from build123d import *

# Parameters (mm, degrees)
SKETCH1_W                               = 304.8
SKETCH1_H                               = 304.8
BOSS_EXTRUDE1_DEPTH                     = 38.1
SKETCH2_R                               = 6.5151
HAAS_T_SLOT_HOLES_DEPTH                 = 219.867836833
SKETCH3_R                               = 9.779
HAAS_COUNTER_BORES_DEPTH                = 22.225
SKETCH4_R                               = 6.5151
TORMACH_T_SLOT_HOLES_DEPTH              = 219.867836833
SKETCH5_R                               = 9.779
TORMACH_COUNTER_BORES_DEPTH             = 22.225
SKETCH6_R                               = 3.0734
SPROCKET_LOCATING_HOLES_DEPTH           = 6.35
SKETCH7_R                               = 3.175
SPROCKET_MOUNTING_CLEARANCE_HOLES_DEPTH = 9.525
SKETCH8_R                               = 5.9182
F_1_2_13_TAPPED_HOLES_DEPTH             = 19.05
SKETCH9_R                               = 3.175
SKETCH9_R_2                             = 3.3
SKETCH9_R_3                             = 2.5
SKETCH9_R_4                             = 4.5
CUT_EXTRUDE1_DEPTH                      = 19.05


with BuildPart() as part:
    # Sketch1 → Boss-Extrude1 (new body)
    with BuildSketch(Plane.XY):
        Rectangle(SKETCH1_W, SKETCH1_H)
    extrude(amount=BOSS_EXTRUDE1_DEPTH)

    # Sketch2 → HAAS T-Slot Holes (cut, through all)
    with BuildSketch(Plane.XY.offset(38.1)):
        with Locations((-127, 101.6)):
            Circle(SKETCH2_R)
        with Locations((127, 101.6)):
            Circle(SKETCH2_R)
        with Locations((127, -101.6)):
            Circle(SKETCH2_R)
        with Locations((-127, -101.6)):
            Circle(SKETCH2_R)
        Circle(SKETCH2_R)
    extrude(amount=-HAAS_T_SLOT_HOLES_DEPTH, mode=Mode.SUBTRACT)

    # Sketch3 → HAAS Counter Bores (cut)
    with BuildSketch(Plane.XY.offset(38.1)):
        with Locations((-127, 101.6)):
            Circle(SKETCH3_R)
        with Locations((127, 101.6)):
            Circle(SKETCH3_R)
        Circle(SKETCH3_R)
        with Locations((127, -101.6)):
            Circle(SKETCH3_R)
        with Locations((-127, -101.6)):
            Circle(SKETCH3_R)
    extrude(amount=-HAAS_COUNTER_BORES_DEPTH, mode=Mode.SUBTRACT)

    # Sketch4 → Tormach T-Slot Holes (cut, through all)
    with BuildSketch(Plane.XY.offset(38.1)):
        with Locations((-101.6, 90.4875)):
            Circle(SKETCH4_R)
        with Locations((101.6, 90.4875)):
            Circle(SKETCH4_R)
        with Locations((-101.6, -90.4875)):
            Circle(SKETCH4_R)
        with Locations((101.6, -90.4875)):
            Circle(SKETCH4_R)
    extrude(amount=-TORMACH_T_SLOT_HOLES_DEPTH, mode=Mode.SUBTRACT)

    # Sketch5 → Tormach Counter bores (cut)
    with BuildSketch(Plane.XY.offset(38.1)):
        with Locations((-101.6, 90.4875)):
            Circle(SKETCH5_R)
        with Locations((101.6, 90.4875)):
            Circle(SKETCH5_R)
        with Locations((101.6, -90.4875)):
            Circle(SKETCH5_R)
        with Locations((-101.6, -90.4875)):
            Circle(SKETCH5_R)
    extrude(amount=-TORMACH_COUNTER_BORES_DEPTH, mode=Mode.SUBTRACT)

    # Sketch6 → Sprocket Locating Holes (cut)
    with BuildSketch(Plane.XY.offset(38.1)):
        with Locations((0, 43.50004)):
            Circle(SKETCH6_R)
        with Locations((0, -43.50004)):
            Circle(SKETCH6_R)
    extrude(amount=-SPROCKET_LOCATING_HOLES_DEPTH, mode=Mode.SUBTRACT)

    # Sketch7 → Sprocket Mounting clearance holes (cut)
    with BuildSketch(Plane.XY.offset(38.1)):
        with Locations((43.50004, 0)):
            Circle(SKETCH7_R)
        with Locations((37.672139706, -21.75002)):
            Circle(SKETCH7_R)
        with Locations((21.75002, -37.672139706)):
            Circle(SKETCH7_R)
        with Locations((-21.75002, -37.672139706)):
            Circle(SKETCH7_R)
        with Locations((-37.672139706, -21.75002)):
            Circle(SKETCH7_R)
        with Locations((-43.50004, 0)):
            Circle(SKETCH7_R)
        with Locations((-37.672139706, 21.75002)):
            Circle(SKETCH7_R)
        with Locations((-21.75002, 37.672139706)):
            Circle(SKETCH7_R)
        with Locations((21.75002, 37.672139706)):
            Circle(SKETCH7_R)
        with Locations((37.672139706, 21.75002)):
            Circle(SKETCH7_R)
    extrude(amount=-SPROCKET_MOUNTING_CLEARANCE_HOLES_DEPTH, mode=Mode.SUBTRACT)

    # Sketch8 → 1/2-13 Tapped Holes (cut)
    with BuildSketch(Plane.XY.offset(38.1)):
        with Locations((-71.4375, 106.4641)):
            Circle(SKETCH8_R)
        with Locations((71.4375, 106.4641)):
            Circle(SKETCH8_R)
        with Locations((71.4375, -106.4641)):
            Circle(SKETCH8_R)
        with Locations((-71.4375, -106.4641)):
            Circle(SKETCH8_R)
    extrude(amount=-F_1_2_13_TAPPED_HOLES_DEPTH, mode=Mode.SUBTRACT)

    # Sketch9 → Cut-Extrude1 (cut)
    with BuildSketch(Plane.XY.offset(38.1)):
        with Locations((106.975954286, 70.395873002)):
            Circle(SKETCH9_R)
        with Locations((106.975954286, 42.900373002)):
            Circle(SKETCH9_R)
        with Locations((8.985545702, 53.468225166)):
            Circle(SKETCH9_R)
        with Locations((41.65587457, 60.657920909)):
            Circle(SKETCH9_R)
        with Locations((-59.73361009, 43.51546635)):
            Circle(SKETCH9_R)
        with Locations((-85.92736009, 17.32171635)):
            Circle(SKETCH9_R)
        with Locations((-59.73361009, -8.87203365)):
            Circle(SKETCH9_R)
        with Locations((-114.633914907, -45.510351778)):
            Circle(SKETCH9_R)
        with Locations((-141.027605333, -76.084724647)):
            Circle(SKETCH9_R_2)
        with Locations((61.148073745, -55.642324401)):
            Circle(SKETCH9_R_2)
        with Locations((23.174346831, -6.319418914)):
            Circle(SKETCH9_R)
        with Locations((60.142975062, 4.412421641)):
            Circle(SKETCH9_R)
        with Locations((50.952707496, -32.969269828)):
            Circle(SKETCH9_R)
        with Locations((-36.264061896, -34.786851156)):
            Circle(SKETCH9_R_3)
        with Locations((-96.280107569, -26.615466331)):
            Circle(SKETCH9_R_3)
        with Locations((-115.245018307, 30.908697539)):
            Circle(SKETCH9_R_3)
        with Locations((-63.965591615, 74.314810953)):
            Circle(SKETCH9_R_3)
        with Locations((-2.610367098, 15.573114042)):
            Circle(SKETCH9_R_3)
        with Locations((14.128233333, 73.914299226)):
            Circle(SKETCH9_R_2)
        with Locations((74.737676016, 34.700608013)):
            Circle(SKETCH9_R_4)
        with Locations((144.776518705, 66.245900326)):
            Circle(SKETCH9_R_4)
        with Locations((122.991918933, 21.088470635)):
            Circle(SKETCH9_R_4)
    extrude(amount=-CUT_EXTRUDE1_DEPTH, mode=Mode.SUBTRACT)


solid = part.part
Geometry check sheet. Reference: the model listing, model coordinates, mm. A direction names the side the tool comes from. Give positions to 0.01 mm unless a question says otherwise; leave off trailing zeros. Write each loop counter-clockwise with the first axis right and the second up, starting at its lowest first coordinate (ties: lowest second). Pieces come first, ordered by that corner, then holes.
1) Cross-section at A-A (x = -127). Record the boundary of the cut face in (y, z) (3 decimals), plus the area to 3 significant figures.
Values follow:
outline: (-152.4, 0) - (-108.115, 0) - (-108.115, 15.875) - (-111.379, 15.875) - (-111.379, 38.1) - (-152.4, 38.1) - close; (-95.085, 0) - (95.085, 0) - (95.085, 15.875) - (91.821, 15.875) - (91.821, 38.1) - (-91.821, 38.1) - (-91.821, 15.875) - (-95.085, 15.875) - close; (108.115, 0) - (152.4, 0) - (152.4, 38.1) - (111.379, 38.1) - (111.379, 15.875) - (108.115, 15.875) - close
area: 10,300 mm2
2) Thickness scan on line 1 (Y direction, x = 101.6, z = 28.5); line 2 (Y direction, x = -127, z = 5); line 3 (Y direction, x = 126, z = 26.5). Record the ranges inside material, lowest first.
Values follow:
line 1: y = -152.4 to -100.27, -80.71 to 80.71, 100.27 to 152.4
line 2: y = -152.4 to -108.12, -95.08 to 95.08, 108.12 to 152.4
line 3: y = -152.4 to -111.33, -91.87 to 17.74, 24.44 to 91.87, 111.33 to 152.4
3) Release check for a two-part mould opening along Y. For faces 3 (the face through (-152.4, -2, 19)), 4 (the face through (71, -106, 19.05)) record: released by +Y, released by -Y, zero draft, split by the parting line, or undercut.
Values follow:
face 3: zero draft
face 4: undercut
4) Go/stop test with flat-tipped pins: pin 1 Ø3 at (x, y) = (10.5, 54) entering from +Z; pin 2 Ø6 at (x, y) = (102, 89.5) entering from +Z; pin 3 Ø1.9 at (x, y) = (38.5, -20.5) entering from +Z (3 decimals). Record where each tip stops, or that it passes through.
Values follow:
pin 1: stops at z = 19.05
pin 2: passes through
pin 3: stops at z = 28.575
5) Set-up check for faces 1 (the face through (-95, -93, 15.875)), 2 (the face through (96.43, -94.45, 8.05)): record each of +Z, -Z, +X, -X, +Y, -Y from which the full face is reachable in a straight line by a thin tool's end or side.
Values follow:
face 1: +Z
face 2: +Z, -Z
